Geometry: final body of the model. Coordinates: model frame, mm. A direction names the side the tool comes from. Give positions to 0.01 mm unless a question says otherwise; leave off trailing zeros. Write each loop counter-clockwise with the first axis right and the second up, starting at its lowest first coordinate (ties: lowest second). Pieces come first, ordered by that corner, then holes. Notation, with made-up numbers: M 49.5,-12 L 73.5,-12 A9 cw 73.5,-6 Z; hole C 5,22 d3. An arc over 180 degrees is marked long. One line per question, with ' | ' between items.
from build123d import *

# Parameters (mm, degrees)
BOSS_EXTRU_1_DEPTH      = 20
ESQUISSE2_W             = 20
ESQUISSE2_H             = 20
BOSS_EXTRU_2_DEPTH      = 4
ESQUISSE3_W             = 20
ESQUISSE3_H             = 20
BOSS_EXTRU_3_DEPTH      = 4
ESQUISSE4_W             = 4
ESQUISSE4_H             = 16
BOSS_EXTRU_4_DEPTH      = 20
CHANFREIN1_SIZE         = 4
ESQUISSE5_R             = 2.1
ENL_V_MAT_EXTRU_1_DEPTH = 36.215222341
ESQUISSE6_R             = 5.5
ENL_V_MAT_EXTRU_2_DEPTH = 32.215222341
D_GAGEMENT_41_D         = 3.4544
D_GAGEMENT_41_DEPTH     = 10
D_GAGEMENT_41_TIP       = 1.037806461
CHANFREIN2_SIZE         = 1.6


with BuildPart() as part:
    # Esquisse1 → Boss.-Extru.1 (new body)
    with BuildSketch(Plane.XY):
        Polygon((0, 0), (0, 20), (17.975880926, 8.767422936), align=None)
    extrude(amount=BOSS_EXTRU_1_DEPTH)

    # Esquisse2 → Boss.-Extru.2 (add)
    with BuildSketch(Plane.ZY):
        with Locations((10, 10)):
            Rectangle(ESQUISSE2_W, ESQUISSE2_H)
    extrude(amount=BOSS_EXTRU_2_DEPTH)

    # Esquisse3 → Boss.-Extru.3 (add)
    with BuildSketch(Plane(origin=(0, 0, 0), x_dir=(0.898794046, 0.438371147, 0), z_dir=(0.438371147, -0.898794046, 0))):
        with Locations((10, 10)):
            Rectangle(ESQUISSE3_W, ESQUISSE3_H)
    extrude(amount=BOSS_EXTRU_3_DEPTH)

    # Esquisse4 → Boss.-Extru.4 (add)
    with BuildSketch(Plane.XY.offset(20)):
        with Locations((-2, 28)):
            Rectangle(ESQUISSE4_W, ESQUISSE4_H)
        Polygon((0, 24), (0, 20), (17.975880926, 8.767422936), (21.571057111, 10.520907523), align=None)
        Polygon((31.215222341, -9.252561496), (21.571057111, 10.520907523), (17.975880926, 8.767422936), (19.729365513, 5.172246751), (27.620046155, -11.006046083), align=None)
        Polygon((0, 0), (-4, 0), (1.753484587, -3.595176185), align=None)
    extrude(amount=-BOSS_EXTRU_4_DEPTH)

    # Chanfrein1
    chanfrein1_edges = [part.edges().sort_by_distance(p)[0] for p in [
        (0, 24, 10),
        (21.571057111, 10.520907523, 10),
    ]]
    chamfer(chanfrein1_edges, length=CHANFREIN1_SIZE)

    # Esquisse5 → Enlèv. mat.-Extru.1 (cut, through all)
    with BuildSketch(Plane.ZY.offset(4)):
        with Locations((10, 28)):
            Circle(ESQUISSE5_R)
    extrude(amount=-ENL_V_MAT_EXTRU_1_DEPTH, mode=Mode.SUBTRACT)

    # Esquisse6 → Enlèv. mat.-Extru.2 (cut, through all)
    with BuildSketch(Plane(origin=(0, 0, 0), x_dir=(0, 0, -1), z_dir=(1, 0, 0))):
        with Locations((-10, 28)):
            Circle(ESQUISSE6_R)
    extrude(amount=ENL_V_MAT_EXTRU_2_DEPTH, mode=Mode.SUBTRACT)

    # Dégagement #41
    with Locations(Plane(origin=(21.571057111, 10.520907523, 0), x_dir=(0, 0, -1), z_dir=(0.898794046, 0.438371147, 0))):
        with Locations((-10, -13)):
            Hole(D_GAGEMENT_41_D / 2, depth=D_GAGEMENT_41_DEPTH)
            with Locations((0, 0, -(D_GAGEMENT_41_DEPTH + D_GAGEMENT_41_TIP / 2))):  # 118° drill point
                Cone(0, D_GAGEMENT_41_D / 2, D_GAGEMENT_41_TIP, mode=Mode.SUBTRACT)

    # Chanfrein2
    chanfrein2_edges = [part.edges().sort_by_distance(p)[0] for p in [
        (0, 36, 10),
        (27.269882019, -1.163415079, 0),
        (31.215222341, -9.252561496, 10),
        (27.269882019, -1.163415079, 20),
        (10.785528556, 17.260453761, 20),
        (10.785528556, 17.260453761, 0),
        (0, 32, 20),
        (0, 32, 0),
        (20.751703212, 9.783157959, 20),
        (20.751703212, 9.783157959, 0),
        (1.696096192, 24.940161472, 20),
        (1.696096192, 24.940161472, 0),
    ]]
    chamfer(chanfrein2_edges, length=CHANFREIN2_SIZE)


solid = part.part
(1) Cut plane D-D, the plane x = 11.5. Return loops of the section in (y, z), then the cut area to 3 significant figures.
Working result:
outline: M 1.16,0 L 14.93,0 L 16.81,1.6 L 16.81,18.4 L 14.93,20 L 1.16,20 Z | area: 310 mm^2
(2) Set-up query: faces 4 (the face through (10.62, 0.73, 10.14)), 5 (the face through (-0.8, 31.7, 19.2)), 6 (the face through (-4, 18, 10)). Return all of +Z, -Z, +X, -X, +Y, -Y with unobstructed straight access to the full face (end or side cutting, diameter ignored); none if empty.
Working result:
face 4: +Z, -Z, -Y | face 5: +Z, +X, +Y | face 6: +Z, -Z, -X, +Y, -Y
(3) First-contact query: P1, Ø3, axis at x = 24.5, z = 9, coming from the -Y side; P2, Ø12, axis at y = 30.5, z = 5, coming from the +X side; P3, Ø1.5, axis at x = 2, z = 8, coming from the -Y side. Flat tips, straight axial feed; report the tip coordinate or a pass-through.
Working result:
P1: stops at y = -7.68 | P2: stops at x = 1.94 | P3: stops at y = -3.6
(4) Cut plane A-A, the plane z = 3.75. Return loops of the section in (x, y), then the cut area to 3 significant figures.
Working result:
outline: M -4,0 L 1.75,-3.6 L 19.73,5.17 L 27.62,-11.01 L 29.78,-9.95 L 30.51,-7.81 L 23.32,6.93 L 18.18,12.64 L 3.39,21.88 L 0,28 L 0,34.4 L -1.6,36 L -4,36 Z | area: 578 mm^2
(5) Material intervals for L1, parallel to X at y = 30, z = 5.5; L2, parallel to Y at x = -1.05, z = 10; L3, parallel to Y at x = 25, z = 9, sorted ascending. Write a range as [from, to].
Working result:
L1: x = [-4, 0] | L2: y = [-1.84, 25.9], [30.1, 35.45] | L3: y = [-5.63, -3.84], [-0.7, 3.49]
(6) Cut plane C-C, the plane z = 10. Return loops of the section in (x, y), then the cut area to 3 significant figures.
Working result:
outline: M -4,0 L 1.75,-3.6 L 19.73,5.17 L 22.92,-1.36 L 26.51,0.39 L 23.32,6.93 L 18.18,12.64 L 3.39,21.88 L 3.05,22.5 L 0,22.5 L 0,25.9 L -4,25.9 Z; M -4,30.1 L 0,30.1 L 0,34.4 L -1.6,36 L -4,36 Z; M 24.43,-4.47 L 27.62,-11.01 L 29.78,-9.95 L 30.51,-7.81 L 28.03,-2.72 Z | area: 539 mm^2
(7) Draft query along Y for faces 1 (the face through (25.414, -1.984, 8.274)), 2 (the face through (7, 9, 0)), 3 (the face through (-3, 36, 10)). Return one class per face: released by +Y, released by -Y, zero draft, split by the parting line, or undercut.
Working result:
face 1: undercut | face 2: zero draft | face 3: released by +Y
(8) Cut plane B-B, the plane y = 3. Return loops of the section in (x, z), then the cut area to 3 significant figures.
Working result:
outline: M -4,0 L 15.28,0 L 15.28,20 L -4,20 Z; M 20.79,0 L 23.46,0 L 25.24,1.6 L 25.24,18.4 L 23.46,20 L 20.79,20 Z | area: 472 mm^2
